Read the model definition and answer for the solid it produces. Units are mm, in the model's axes. A direction names the side the tool comes from. Coordinates: 2 decimals unless noted, no trailing zeros. Order: outer loops, then holes, each group sorted by start corner. A loop starts at its lowest first (then second) coordinate and runs counter-clockwise, first axis right, second up.
```python
from build123d import *

# Parameters (mm, degrees)
SKETCH1_W           = 40
SKETCH1_H           = 40
BOSS_EXTRUDE1_DEPTH = 40
CUT_EXTRUDE1_DEPTH  = 40
SKETCH3_W           = 20
SKETCH3_H           = 20
CUT_EXTRUDE2_DEPTH  = 40
CUT_EXTRUDE4_DEPTH  = 20


with BuildPart() as part:
    # Sketch1 → Boss-Extrude1 (new body)
    with BuildSketch(Plane.XY):
        with Locations((20, 20)):
            Rectangle(SKETCH1_W, SKETCH1_H)
    extrude(amount=BOSS_EXTRUDE1_DEPTH)

    # Sketch2 → Cut-Extrude1 (cut)
    with BuildSketch(Plane.XY.offset(40)):
        Polygon((40, 40), (0, 40), (0, 20), align=None)
    extrude(amount=-CUT_EXTRUDE1_DEPTH, mode=Mode.SUBTRACT)

    # Sketch3 → Cut-Extrude2 (cut)
    with BuildSketch(Plane(origin=(40, 0, 0), x_dir=(0, 0, -1), z_dir=(1, 0, 0))):
        with Locations((-30, 30)):
            Rectangle(SKETCH3_W, SKETCH3_H)
    extrude(amount=-CUT_EXTRUDE2_DEPTH, mode=Mode.SUBTRACT)

    # Sketch4 → Cut-Extrude4 (cut)
    with BuildSketch(Plane.XY.offset(40)):
        Polygon((0, 20), (20, 0), (0, 0), align=None)
    extrude(amount=-CUT_EXTRUDE4_DEPTH, mode=Mode.SUBTRACT)


solid = part.part
```
1) Flat-ended cylindrical pins translate along their axes: pin 1 Ø10 at (x, z) = (19.5, 15.5) entering from +Y; pin 2 Ø5 at (y, z) = (16.5, 33) entering from -X; pin 3 Ø5 at (x, z) = (8.5, 14) entering from +Y. Find the tip coordinate at first contact, or state that the pin passes through.
A:
pin 1: stops at y = 32.25
pin 2: stops at x = 1
pin 3: stops at y = 25.5
2) Straight lines are drawn through the part: line 1 (Y direction, x = 35, z = 28.5); line 2 (X direction, y = 9, z = 30). For each, find the intervals that lie inside material, in ascending order.
A:
line 1: y = 0 to 20
line 2: x = 11 to 40
3) Which of the six approach directions +Z, -Z, +X, -X, +Y, -Y give full straight-line access (tool end or side, diameter ignored) to faces 1 (the flat face through (6, 6, 20)), 2 (the flat face through (20, 20, 30)), 3 (the flat face through (0, 10, 10))?
A:
face 1: +Z, -X, -Y
face 2: +Z, +X, -X, +Y
face 3: +Z, -Z, -X, +Y, -Y
4) A cutting plane is placed at D-D, the plane x = 33.5. Determine the outline of the cut face in (y, z), and give its area (4 significant figures).
A:
outline: (0, 0) - (36.75, 0) - (36.75, 20) - (20, 20) - (20, 40) - (0, 40) - close
area: 1,135 mm2
5) A cutting plane is placed at A-A, the plane x = 3. Determine the outline of the cut face in (y, z).
A:
outline: (0, 0) - (21.5, 0) - (21.5, 20) - (20, 20) - (20, 40) - (17, 40) - (17, 20) - (0, 20) - close
6) A cutting plane is placed at B-B, the plane y = 15.5. Determine the outline of the cut face in (x, z).
A:
outline: (0, 0) - (40, 0) - (40, 40) - (4.5, 40) - (4.5, 20) - (0, 20) - close
7) A cutting plane is placed at C-C, the plane z = 26. Determine the outline of the cut face in (x, y), and give its area (3 significant figures).
A:
outline: (0, 20) - (20, 0) - (40, 0) - (40, 20) - close
area: 600 mm2
